Answer from the drawing. Dimensions are ordinates in mm from the lowest x, y and z of the part. A direction names the side the tool comes from. Coordinates: 2 decimals unless noted, no trailing zeros. Loops run counter-clockwise (first coordinate to the right, second up) from the corner with the lowest first, then second, coordinate; pieces in that order, holes last.
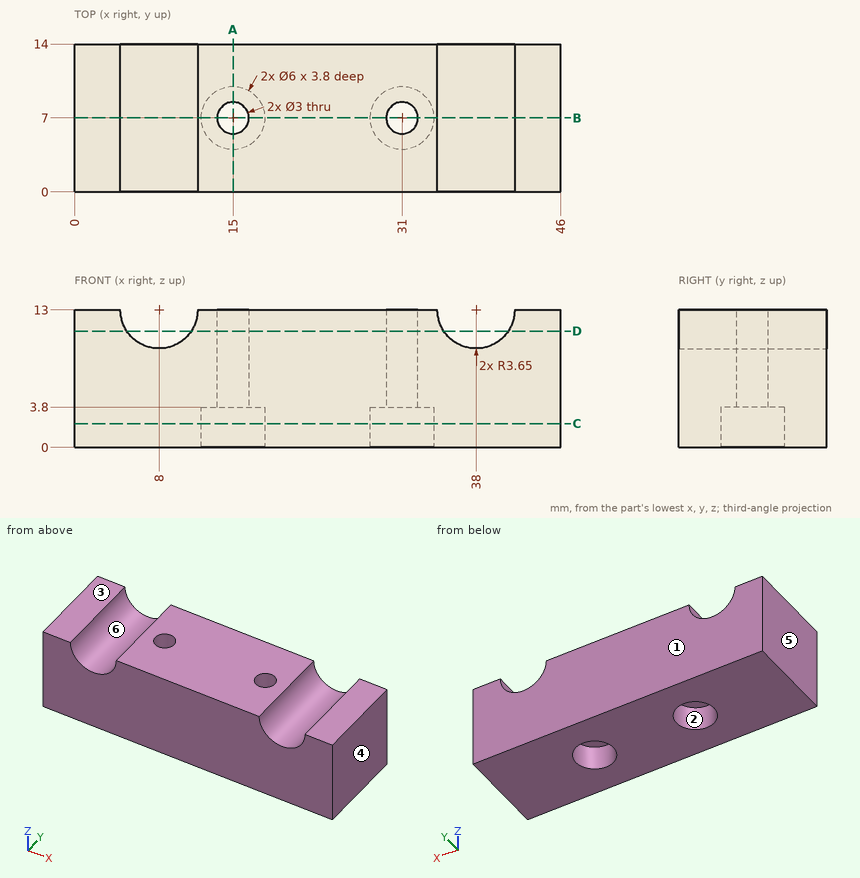
Item 1: Find the intervals of material crossed by line 1 along Y through (x, z) = (31, 1.6); line 2 along Y through (x, z) = (15, 6.75); line 3 along X through (y, z) = (8.75, 12.5), in increasing order.
Numbers:
line 1: y = 0 to 4, 10 to 14
line 2: y = 0 to 5.5, 8.5 to 14
line 3: x = 0 to 4.38, 11.62 to 34.38, 41.62 to 46
Item 2: A cutting plane is placed at A-A on x = 15. Determine the outline of the cut face in (y, z).
Numbers:
outline: (0, 0) - (4, 0) - (4, 3.8) - (5.5, 3.8) - (5.5, 13) - (0, 13) - close; (8.5, 3.8) - (10, 3.8) - (10, 0) - (14, 0) - (14, 13) - (8.5, 13) - close
Item 3: A cutting plane is placed at D-D on z = 11. Determine the outline of the cut face in (x, y).
Numbers:
outline: (0, 0) - (4.95, 0) - (4.95, 14) - (0, 14) - close; (11.05, 0) - (34.95, 0) - (34.95, 14) - (11.05, 14) - close; (41.05, 0) - (46, 0) - (46, 14) - (41.05, 14) - close; hole circle Ø3 at (15, 7); hole circle Ø3 at (31, 7)
Item 4: Determine the mould class of the marked faces 3, 4, 5 and 6 for opening direction X: released by +X, released by -X, zero draft, split by the parting line, or undercut.
Numbers:
face 3: zero draft
face 4: released by +X
face 5: released by -X
face 6: undercut
Item 5: A cutting plane is placed at B-B on y = 7. Determine the outline of the cut face in (x, z), then the cut area to 3 significant figures.
Numbers:
outline: (0, 0) - (12, 0) - (12, 3.8) - (13.5, 3.8) - (13.5, 13) - (11.65, 13) arc R3.65 cw to (4.35, 13) - (0, 13) - close; (16.5, 3.8) - (18, 3.8) - (18, 0) - (28, 0) - (28, 3.8) - (29.5, 3.8) - (29.5, 13) - (16.5, 13) - close; (32.5, 3.8) - (34, 3.8) - (34, 0) - (46, 0) - (46, 13) - (41.65, 13) arc R3.65 cw to (34.35, 13) - (32.5, 13) - close
area: 455 mm2
Item 6: Which of the six approach directions +Z, -Z, +X, -X, +Y, -Y give full straight-line access (tool end or side, diameter ignored) to the marked faces 1 and 2?
Numbers:
face 1: +Z, -Z, +X, -X, +Y
face 2: -Z
Item 7: Given pin 1 (1.8 mm diameter, centred on x = 31, y = 6, fed in from -Z), flat-ended and moving along its own axis, determine where the tip first touches the part or whether it passes through.
Numbers:
pin 1: stops at z = 3.8
Item 8: A cutting plane is placed at C-C on z = 2.25. Determine the outline of the cut face in (x, y), then the cut area to 3 significant figures.
Numbers:
outline: (0, 0) - (46, 0) - (46, 14) - (0, 14) - close; hole circle Ø6 at (15, 7); hole circle Ø6 at (31, 7)
area: 587 mm2
